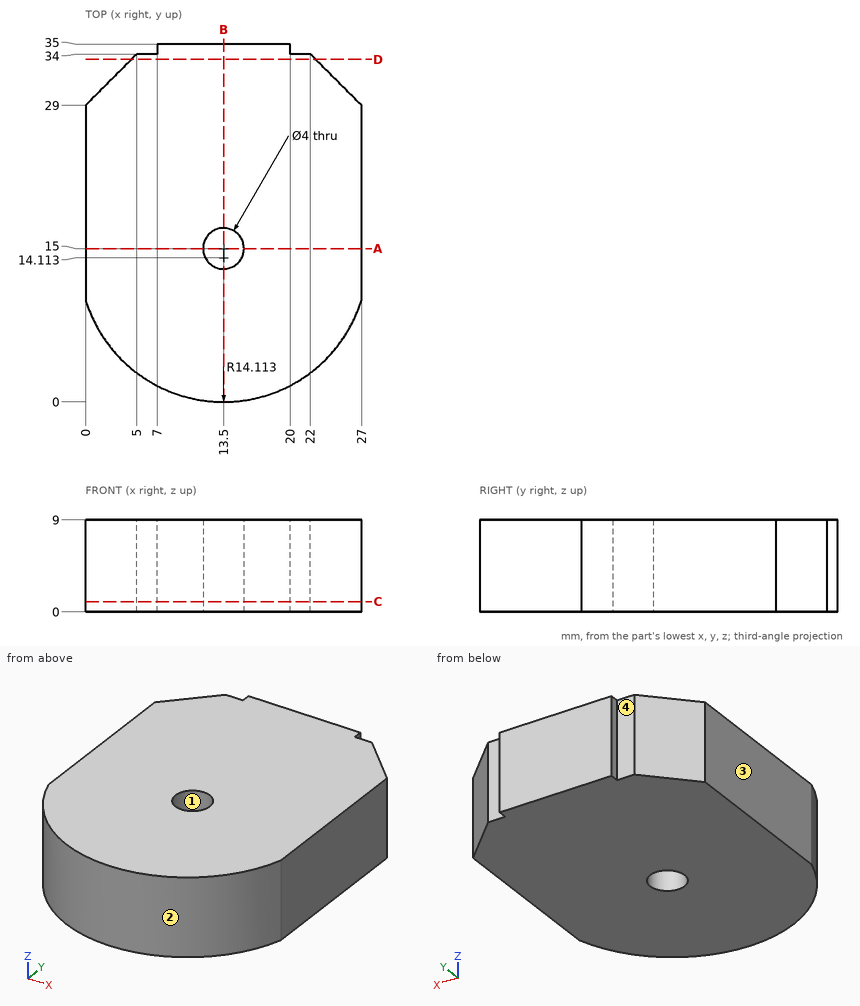
For this review, use the dimensioned drawing (mm, ordinates from the lowest corner) and the shaded views. Round coordinates to 2 decimals unless told otherwise and drop trailing zeros. Write each loop counter-clockwise with the first axis right and the second up, starting at its lowest first coordinate (ties: lowest second). Pieces come first, ordered by that corner, then holes. Notation, with made-up numbers: (32.25, 3.5) - (63.25, 3.5) arc R36 cw to (63.25, 42.5) - close; hole circle Ø9 at (83, 79). An arc over 180 degrees is marked (long way). Answer as a JSON object with one key per item and string values.
1. We need section D-D on y = 33.5. Give the boundary of the cut face in (x, z).
Response values:
{"outline": "(4.5, 0) - (22.5, 0) - (22.5, 9) - (4.5, 9) - close"}
2. We need section A-A on y = 15. Give the boundary of the cut face in (x, z).
Response values:
{"outline": "(0, 0) - (11.5, 0) - (11.5, 9) - (0, 9) - close; (15.5, 0) - (27, 0) - (27, 9) - (15.5, 9) - close"}
3. We need section C-C on z = 1. Give the boundary of the cut face in (x, y) (1 decimal), then the cut area to 3 significant figures.
Response values:
{"outline": "(0, 10) arc R14.1 ccw to (27, 10) - (27, 29) - (22, 34) - (20, 34) - (20, 35) - (7, 35) - (7, 34) - (5, 34) - (0, 29) - close; hole circle Ø4 at (13.5, 15)", "area": "822 mm2"}
4. To check wall thickness, follow line 1 along Y through (x, z) = (12.5, 0.75) (1 decimal); line 2 along X through (y, z) = (16, 1); line 3 along Y through (x, z) = (12.75, 6.25) (1 decimal). State the ranges of each line that lie inside material, in increasing order.
Response values:
{"line 1": "y = 0 to 13.3, 16.7 to 35", "line 2": "x = 0 to 11.77, 15.23 to 27", "line 3": "y = 0 to 13.1, 16.9 to 35"}
5. For pin 1 Ø2 at (x, y) = (23, 16.5) entering from -Z; pin 2 Ø0.8 at (y, z) = (34.5, 2.5) entering from -X; pin 3 Ø3 at (x, z) = (4, 1.5) entering from +Y; pin 4 Ø0.5 at (y, z) = (34.5, 3) entering from +X, all flat-tipped, find the tip position at first contact; note any pin that passes through.
Response values:
{"pin 1": "stops at z = 0", "pin 2": "stops at x = 7", "pin 3": "stops at y = 34", "pin 4": "stops at x = 20"}
6. Draft analysis for pull direction Y (two halves, no side actions). For the marked faces 1, 2, 3 and 4, state which applies: +Y half, -Y half, draft (parallel to the pull), parting line (faces both ways), or undercut.
Response values:
{"face 1": "undercut", "face 2": "-Y half", "face 3": "draft", "face 4": "+Y half"}
7. We need section B-B on x = 13.5. Give the boundary of the cut face in (y, z), then the cut area to 3 significant figures.
Response values:
{"outline": "(0, 0) - (13, 0) - (13, 9) - (0, 9) - close; (17, 0) - (35, 0) - (35, 9) - (17, 9) - close", "area": "279 mm2"}
